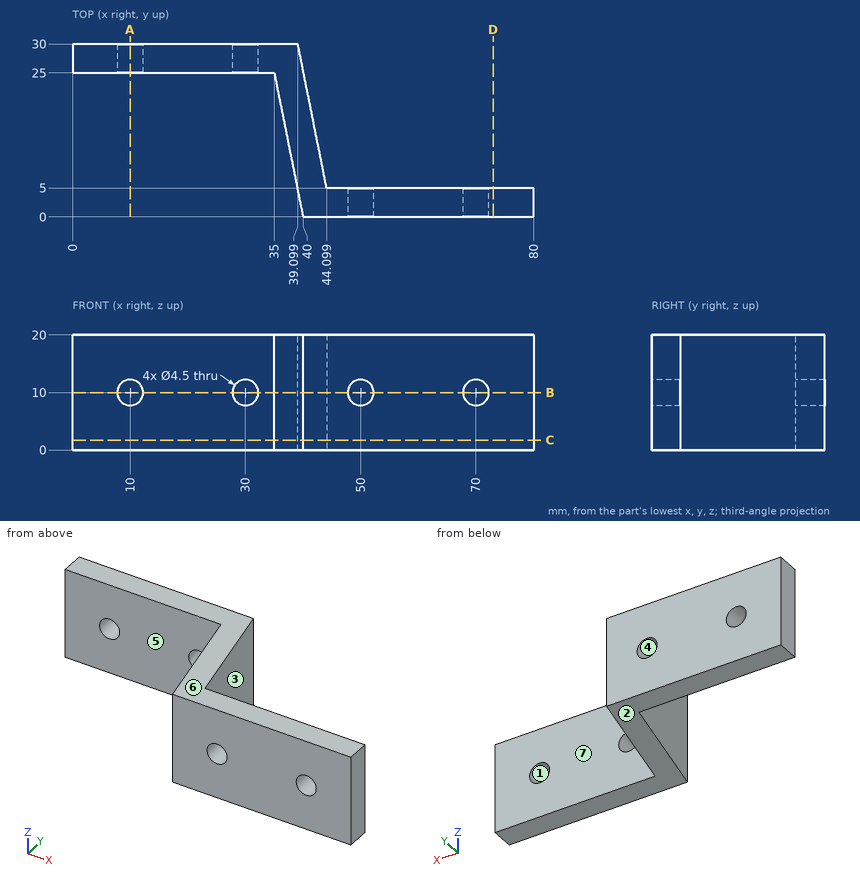
Can you work these out from the drawing? Everything is in mm from the part's minimum corner. A direction names the side the tool comes from. Round coordinates to 2 decimals unless told otherwise and drop trailing zeros. Loops run counter-clockwise (first coordinate to the right, second up) from the corner with the lowest first, then second, coordinate; pieces in that order, holes last. Notation, with made-up numbers: (15.5, 53.5) - (39.5, 53.5) arc R26 ccw to (39.5, 87.5) - close; hole circle Ø11 at (89, 3.25). An arc over 180 degrees is marked (long way). One line per question, with ' | ' between items. Start each with the question number.
Q1. For the marked faces 5, 6 and 7, which set-ups out of +Z, -Z, +X, -X, +Y, -Y let a thin tool reach every point of the face, with its end or its side?
Q2. We'd pull the mould along X, two halves only. Please class the marked faces 1, 2, 3 and 4: +X half, -X half, draft (parallel to the pull), parting line (faces both ways), or undercut.
Q3. I want a section at B-B (z = 10). Write out the boundary of the cut face in (x, y).
Q4. Please list where these lines run through material, in increasing order: line 1 (Z direction, x = 50, y = 1); line 2 (Y direction, x = 55, z = 13.75); line 3 (Y direction, x = 17, z = 13.25). Write a range as [from, to].
Q5. I want a section at A-A (x = 10). Write out the boundary of the cut face in (y, z), then the cut area to 3 significant figures.
Q6. I want a section at C-C (z = 1.75). Write out the boundary of the cut face in (x, y), then the cut area to 3 significant figures.
Q7. I want a section at D-D (x = 73). Write out the boundary of the cut face in (y, z).
Q8. Will these pins go through, and if not, where does the flat tip stop? pin 1 (6 mm diameter, centred on x = 64.5, z = 13.5, fed in from +Y); pin 2 (4 mm diameter, centred on y = 24.5, z = 3.5, fed in from +X); pin 3 (8 mm diameter, centred on y = 26, z = 14, fed in from -X); pin 4 (5 mm diameter, centred on x = 10, z = 10, fed in from -Y).
Response values:
1) face 5: +Z, -Z, -X, -Y | face 6: +Z, +X, -X, +Y, -Y | face 7: +Z, -Z, +X, +Y
2) face 1: undercut | face 2: draft | face 3: +X half | face 4: undercut
3) outline: (0, 25) - (7.75, 25) - (7.75, 30) - (0, 30) - close; (12.25, 25) - (27.75, 25) - (27.75, 30) - (12.25, 30) - close; (32.25, 25) - (35, 25) - (40, 0) - (47.75, 0) - (47.75, 5) - (44.1, 5) - (39.1, 30) - (32.25, 30) - close; (52.25, 0) - (67.75, 0) - (67.75, 5) - (52.25, 5) - close; (72.25, 0) - (80, 0) - (80, 5) - (72.25, 5) - close
4) line 1: z = [0, 7.75], [12.25, 20] | line 2: y = [0, 5] | line 3: y = [25, 30]
5) outline: (25, 0) - (30, 0) - (30, 7.75) - (25, 7.75) - close; (25, 12.25) - (30, 12.25) - (30, 20) - (25, 20) - close | area: 77.5 mm²
6) outline: (0, 25) - (35, 25) - (40, 0) - (80, 0) - (80, 5) - (44.1, 5) - (39.1, 30) - (0, 30) - close | area: 502 mm²
7) outline: (0, 0) - (5, 0) - (5, 20) - (0, 20) - close
8) pin 1: stops at y = 5 | pin 2: stops at x = 40.6 | pin 3: stops at x = 0 | pin 4: stops at y = 25
